Here's how the part is built. I have some questions about the finished solid (model axes, mm). Face numbers are marked on the shaded views. Give positions to 0.01 mm unless a question says otherwise; leave off trailing zeros. Write each loop counter-clockwise with the first axis right and the second up, starting at its lowest first coordinate (ties: lowest second). Pieces come first, ordered by that corner, then holes. Notation, with made-up numbers: (-36.5, 21.25) - (21.5, 21.25) arc R28 cw to (21.5, 42.25) - close; hole circle Ø3 at (72, 55.25). An arc over 180 degrees is marked (long way). Use a Markdown table: item, result.
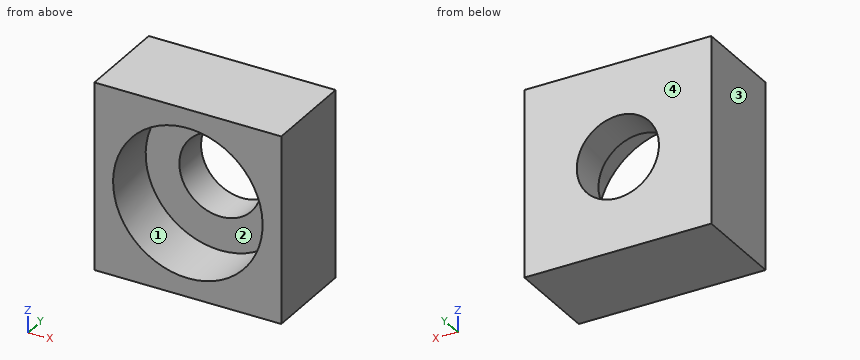
```python
from build123d import *

# Parameters (mm, degrees)
SKETCH1_W           = 10
SKETCH1_H           = 10
SKETCH1_R           = 4
SKETCH1_R_2         = 2.2
BOSS_EXTRUDE1_DEPTH = 5
SKETCH3_R           = 4
SKETCH3_R_2         = 2.2
CUT_EXTRUDE3_DEPTH  = 3


with BuildPart() as part:
    # Sketch1 → Boss-Extrude1 (new body)
    with BuildSketch(Plane(origin=(0, 0, 0), x_dir=(1, 0, 0), z_dir=(0, 1, 0))):
        Rectangle(SKETCH1_W, SKETCH1_H)
        Circle(SKETCH1_R, mode=Mode.SUBTRACT)
        Circle(SKETCH1_R)
        with Locations(Location((0, 0, 0), (0, 0, 270))):
            Circle(SKETCH1_R_2, mode=Mode.SUBTRACT)
    extrude(amount=BOSS_EXTRUDE1_DEPTH)

    # Sketch3 → Cut-Extrude3 (cut)
    with BuildSketch(Plane.XZ):
        with Locations(Location((0, 0, 0), (0, 0, 270))):
            Circle(SKETCH3_R)
        with Locations(Location((0, 0, 0), (0, 0, 270))):
            Circle(SKETCH3_R_2, mode=Mode.SUBTRACT)
    extrude(amount=-CUT_EXTRUDE3_DEPTH, mode=Mode.SUBTRACT)


solid = part.part
```
Item 1: Thinking about a two-plate mould opening in X: for the marked faces 1, 2, 3 and 4, which applies, +X half, -X half, draft (parallel to the pull), parting line (faces both ways), or undercut?
Values:
| item | result |
|---|---|
| face 1 | undercut |
| face 2 | undercut |
| face 3 | -X half |
| face 4 | draft |
Item 2: I need wall thicknesses on line 1 along X through (y, z) = (0.8, 0); line 2 along Z through (x, y) = (0, 4.3). Which ranges of each line are inside material? Lowest first, please. Write a range as [from, to].
Values:
| item | result |
|---|---|
| line 1 | x = [-5, -4], [4, 5] |
| line 2 | z = [-5, -2.2], [2.2, 5] |
Item 3: If we section it at D-D, the plane z = 3.5: Write out the boundary of the cut face in (x, y).
Values:
| item | result |
|---|---|
| outline | (-5, 0) - (-1.94, 0) - (-1.94, 3) - (1.94, 3) - (1.94, 0) - (5, 0) - (5, 5) - (-5, 5) - close |
Item 4: If we section it at A-A, the plane z = 0: Write out the boundary of the cut face in (x, y), plus the area to 3 significant figures.
Values:
| item | result |
|---|---|
| outline | (-5, 0) - (-4, 0) - (-4, 3) - (-2.2, 3) - (-2.2, 5) - (-5, 5) - close; (2.2, 3) - (4, 3) - (4, 0) - (5, 0) - (5, 5) - (2.2, 5) - close |
| area | 17.2 mm2 |
Item 5: If we section it at B-B, the plane y = 0.4: Write out the boundary of the cut face in (x, z), plus the area to 3 significant figures.
Values:
| item | result |
|---|---|
| outline | (-5, -5) - (5, -5) - (5, 5) - (-5, 5) - close; hole circle Ø8 at (0, 0) |
| area | 49.7 mm2 |
Item 6: If we section it at C-C, the plane x = -1: Write out the boundary of the cut face in (y, z).
Values:
| item | result |
|---|---|
| outline | (0, -5) - (5, -5) - (5, -1.96) - (3, -1.96) - (3, -3.87) - (0, -3.87) - close; (0, 3.87) - (3, 3.87) - (3, 1.96) - (5, 1.96) - (5, 5) - (0, 5) - close |
Item 7: Will these pins go through, and if not, where does the flat tip stop? pin 1 Ø5 at (x, z) = (-3.5, -1) entering from -Y; pin 2 Ø5.5 at (x, z) = (0, 0) entering from -Y.
Values:
| item | result |
|---|---|
| pin 1 | stops at y = 0 |
| pin 2 | stops at y = 3 |
